Part print with two shaded views. Sizes in mm from the minimum x, y, z corner. Round coordinates to 2 decimals unless told otherwise and drop trailing zeros. Order: outer loops, then holes, each group sorted by start corner. A loop starts at its lowest first (then second) coordinate and runs counter-clockwise, first axis right, second up. Notation, with made-up numbers: (1, 66) - (53, 66) arc R7 ccw to (53, 75) - close; hole circle Ø10 at (76.25, -20.75). An arc over 180 degrees is marked (long way). Write item = value, one per line.
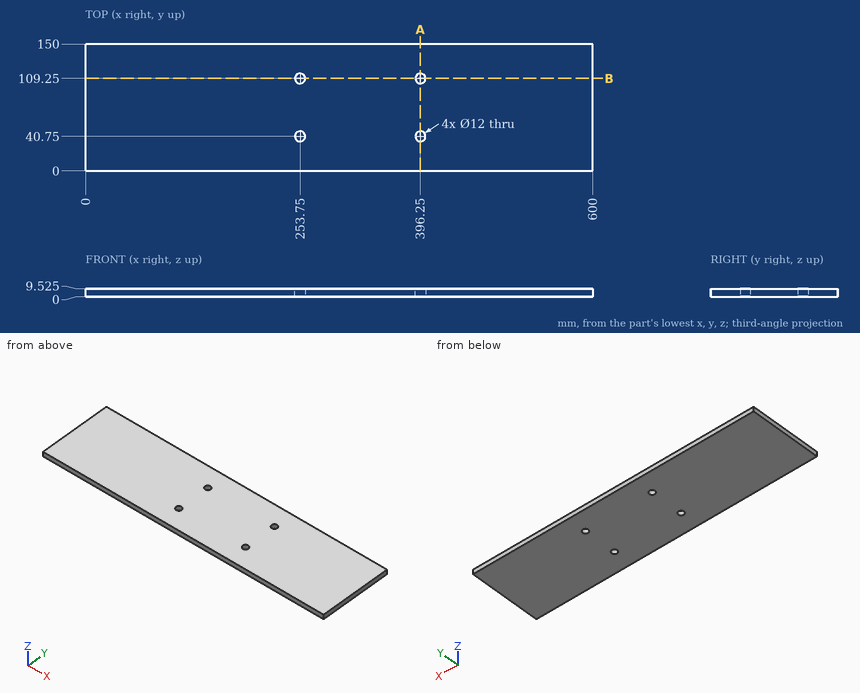
1) Cut at A-A (x = 396.25). Write the cut outline in (y, z) (3 decimals).
Conclusion:
outline = (0, 0) - (34.75, 0) - (34.75, 9.525) - (0, 9.525) - close; (46.75, 0) - (103.25, 0) - (103.25, 9.525) - (46.75, 9.525) - close; (115.25, 0) - (150, 0) - (150, 9.525) - (115.25, 9.525) - close
2) Cut at B-B (y = 109.25). Write the cut outline in (x, z) (3 decimals).
Conclusion:
outline = (0, 0) - (247.75, 0) - (247.75, 9.525) - (0, 9.525) - close; (259.75, 0) - (390.25, 0) - (390.25, 9.525) - (259.75, 9.525) - close; (402.25, 0) - (600, 0) - (600, 9.525) - (402.25, 9.525) - close
3) Wall check: line 1 along Y through (x, z) = (253.75, 4.5); line 2 along X through (y, z) = (40.75, 5.5); line 3 along Y through (x, z) = (249, 1). Give the ranges that are in metal, low to high.
Conclusion:
line_1 = 0 to 34.75, 46.75 to 103.25, 115.25 to 150
line_2 = 0 to 247.75, 259.75 to 390.25, 402.25 to 600
line_3 = 0 to 37.08, 44.42 to 105.58, 112.92 to 150
